from build123d import *

# Parameters (mm, degrees)
SKETCH1_W           = 59
SKETCH1_H           = 43
BOSS_EXTRUDE1_DEPTH = 3
SKETCH2_R           = 5
BOSS_EXTRUDE2_DEPTH = 17
SKETCH3_W           = 17
SKETCH3_H           = 11
BOSS_EXTRUDE3_DEPTH = 7
SKETCH4_W           = 5.5
SKETCH4_H           = 15
BOSS_EXTRUDE4_DEPTH = 7
FILLET1_R           = 5
SKETCH5_W           = 7.5
SKETCH5_H           = 6
SKETCH5_W_2         = 10
BOSS_EXTRUDE5_DEPTH = 10
SKETCH6_W           = 6
SKETCH6_H           = 10.2
BOSS_EXTRUDE6_DEPTH = 12
SKETCH7_W           = 10
SKETCH7_H           = 25
BOSS_EXTRUDE7_DEPTH = 8
CHAMFER1_SIZE       = 1.5
SKETCH8_W           = 6
SKETCH8_H           = 6
BOSS_EXTRUDE8_DEPTH = 5
SKETCH9_R           = 1.85
BOSS_EXTRUDE9_DEPTH = 1.5


with BuildPart() as part:
    # Sketch1 → Boss-Extrude1 (new body)
    with BuildSketch(Plane(origin=(0, 0, 0), x_dir=(1, 0, 0), z_dir=(0, 1, 0))):
        Rectangle(SKETCH1_W, SKETCH1_H)
    extrude(amount=BOSS_EXTRUDE1_DEPTH)

    # Sketch2 → Boss-Extrude2 (add)
    with BuildSketch(Plane(origin=(0, 3, 0), x_dir=(1, 0, 0), z_dir=(0, 1, 0))):
        with Locations(Location((-21.5, 15.5, 0), (0, 0, 90))):
            Circle(SKETCH2_R)
    extrude(amount=BOSS_EXTRUDE2_DEPTH)

    # Sketch3 → Boss-Extrude3 (add)
    with BuildSketch(Plane(origin=(0, 3, 0), x_dir=(1, 0, 0), z_dir=(0, 1, 0))):
        with Locations((-27.5, -14)):
            Rectangle(SKETCH3_W, SKETCH3_H)
    extrude(amount=BOSS_EXTRUDE3_DEPTH)

    # Sketch4 → Boss-Extrude4 (add)
    with BuildSketch(Plane(origin=(0, 3, 0), x_dir=(1, 0, 0), z_dir=(0, 1, 0))):
        with Locations((20.25, 19)):
            Rectangle(SKETCH4_W, SKETCH4_H)
    extrude(amount=BOSS_EXTRUDE4_DEPTH)

    # Fillet1
    fillet1_edges = [part.edges().sort_by_distance(p)[0] for p in [
        (-21.5, 20, -10.5),
    ]]
    fillet(fillet1_edges, radius=FILLET1_R)

    # Sketch5 → Boss-Extrude5 (add)
    with BuildSketch(Plane(origin=(0, 3, 0), x_dir=(1, 0, 0), z_dir=(0, 1, 0))):
        with Locations((-5.25, -16.5)):
            Rectangle(SKETCH5_W, SKETCH5_H)
        with Locations((7.5, 12.5)):
            Rectangle(SKETCH5_W_2, SKETCH5_H)
        with Locations((7.5, 0)):
            Rectangle(SKETCH5_W_2, SKETCH5_H)
        with Locations((7.5, -8.5)):
            Rectangle(SKETCH5_W_2, SKETCH5_H)
    extrude(amount=BOSS_EXTRUDE5_DEPTH)

    # Sketch6 → Boss-Extrude6 (add)
    with BuildSketch(Plane(origin=(0, 3, 0), x_dir=(1, 0, 0), z_dir=(0, 1, 0))):
        with Locations((-25, 2)):
            Rectangle(SKETCH6_W, SKETCH6_H)
    extrude(amount=BOSS_EXTRUDE6_DEPTH)

    # Sketch7 → Boss-Extrude7 (add)
    with BuildSketch(Plane(origin=(0, 3, 0), x_dir=(1, 0, 0), z_dir=(0, 1, 0))):
        with Locations((-6.5, 4)):
            Rectangle(SKETCH7_W, SKETCH7_H)
    extrude(amount=BOSS_EXTRUDE7_DEPTH)

    # Chamfer1
    chamfer1_edges = [part.edges().sort_by_distance(p)[0] for p in [
        (-1.5, 11, -4),
        (-11.5, 11, -4),
    ]]
    chamfer(chamfer1_edges, length=CHAMFER1_SIZE)

    # Sketch8 → Boss-Extrude8 (add)
    with BuildSketch(Plane(origin=(0, 3, 0), x_dir=(1, 0, 0), z_dir=(0, 1, 0))):
        with Locations((-15, 6.5)):
            Rectangle(SKETCH8_W, SKETCH8_H)
    extrude(amount=BOSS_EXTRUDE8_DEPTH)

    # Sketch9 → Boss-Extrude9 (add)
    with BuildSketch(Plane(origin=(0, 8, 0), x_dir=(1, 0, 0), z_dir=(0, 1, 0))):
        with Locations(Location((-15, 6.5, 0), (0, 0, 90))):
            Circle(SKETCH9_R)
    extrude(amount=BOSS_EXTRUDE9_DEPTH)


solid = part.part
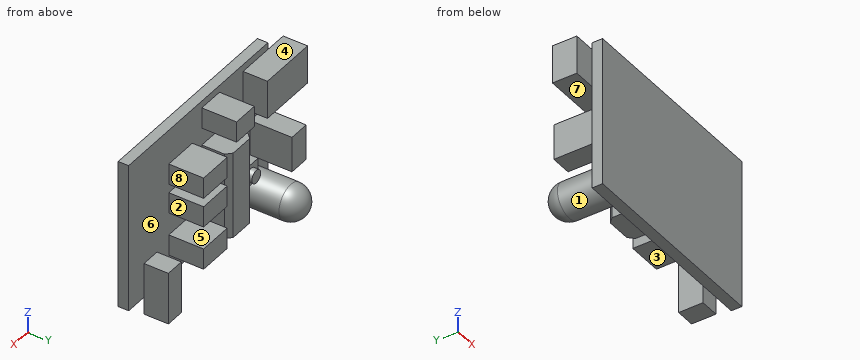
Can you work these out from the model? Positions are in its coordinate system, mm. Face numbers are marked on the shaded views. A direction names the side the tool comes from. Give positions to 0.01 mm unless a question says otherwise; leave off trailing zeros. Write each loop counter-clockwise with the first axis right and the second up, starting at its lowest first coordinate (ties: lowest second). Pieces come first, ordered by that corner, then holes. Notation, with made-up numbers: (-36.5, 21.5) -> (13.5, 21.5) arc R31 cw to (13.5, 60.5) -> close; hole circle Ø7 at (12, -35). An arc over 180 degrees is marked (long way). Answer as a JSON object with one key per item and string values. Group by question number.
Item 1: For the marked faces 1, 2, 3, 4 and 5, which set-ups out of +Z, -Z, +X, -X, +Y, -Y let a thin tool reach every point of the face, with its end or its side?
Item 2: Suppose I cut it at C-C (z = -6). Please give me the cut outline in (x, y), plus the area to 3 significant figures.
Item 3: Suppose I cut it at D-D (x = -15). Please give me the cut outline in (y, z).
Item 4: Please list where these lines run through material, in increasing order: line 1 (X direction, y = 4.5, z = -6.5); line 2 (X direction, y = 6.25, z = 7); line 3 (X direction, y = 9.25, z = 16). Write a range as [from, to].
Item 5: Suppose I cut it at A-A (x = 5). Please give me the cut outline in (y, z).
Item 6: Suppose I cut it at B-B (y = 4). State how many separate pieces and enclosed holes the cut face has, plus the area to 3 significant figures.
Item 7: I'm going to push flat-ended pins straight in: P1, Ø1, axis at x = 1, z = 8, coming from the +Y side; P2, Ø3, axis at x = -25.5, y = 9.5, coming from the -Z side; P3, Ø2.5, axis at x = 21, z = -23.5, coming from the -Y side. Where does each tip first touch, or does it pass through?
Item 8: We'd pull the mould along X, two halves only. Please class the marked faces 6, 7 and 8: +X half, -X half, draft (parallel to the pull), parting line (faces both ways), or undercut.
Findings:
{
 "1": {"face 1": "+Y", "face 2": "+Z, -Z, +X, +Y", "face 3": "-Z, +Y", "face 4": "+Z, +X, -X, +Y", "face 5": "+X, +Y"},
 "2": {"outline": "(-29.5, 0) -> (29.5, 0) -> (29.5, 3) -> (-1.5, 3) -> (-1.5, 9.5) -> (-3, 11) -> (-10, 11) -> (-11.5, 9.5) -> (-11.5, 3) -> (-12, 3) -> (-12, 8) -> (-13.22, 8) -> (-13.22, 9.5) -> (-16.78, 9.5) -> (-16.78, 8) -> (-18, 8) -> (-18, 3) -> (-22, 3) -> (-22, 15) -> (-28, 15) -> (-28, 3) -> (-29.5, 3) -> close", "area": "362 mm²"},
 "3": {"outline": "(0, -21.5) -> (3, -21.5) -> (3, -9.5) -> (8, -9.5) -> (8, -8.35) -> (9.5, -8.35) -> (9.5, -4.65) -> (8, -4.65) -> (8, -3.5) -> (3, -3.5) -> (3, 21.5) -> (0, 21.5) -> close"},
 "4": {"line 1": "x = [-28, -22], [-18, -12], [-11.5, -1.5]", "line 2": "x = [-11.5, -1.5], [2.5, 12.5]", "line 3": "x = [-36, -19], [-9, -1.5]"},
 "5": {"outline": "(0, -21.5) -> (3, -21.5) -> (3, -15.5) -> (13, -15.5) -> (13, -9.5) -> (3, -9.5) -> (3, -3) -> (13, -3) -> (13, 3) -> (3, 3) -> (3, 5.5) -> (13, 5.5) -> (13, 11.5) -> (3, 11.5) -> (3, 21.5) -> (0, 21.5) -> close"},
 "6": {"separate pieces": "10", "enclosed holes": "0", "area": "920 mm²"},
 "7": {"P1": "stops at y = 3", "P2": "stops at z = -19.83", "P3": "stops at y = 3"},
 "8": {"face 6": "undercut", "face 7": "draft", "face 8": "+X half"}
}
